Drawing for the job (mm, zero at the part's lowest x, y, z). Coordinates: 2 decimals unless noted, no trailing zeros. Order: outer loops, then holes, each group sorted by start corner. A loop starts at its lowest first (then second) coordinate and runs counter-clockwise, first axis right, second up.
1) Cut at A-A (y = 57.15). List the corners of the cut face in (x, z) (3 decimals), and give its area (3 significant figures).
2) Cut at D-D (z = 152). List the corners of the cut face in (x, y) (3 decimals).
3) Cut at B-B (z = 20). List the corners of the cut face in (x, y) (3 decimals).
4) Mould opens along X. For the marked faces 1, 2 and 3 say: +X half, -X half, draft (parallel to the pull), parting line (faces both ways), or undercut.
5) Pin check, flat tips, straight feed: pin 1 Ø1.5 at (y, z) = (34, 126.5) entering from -X; pin 2 Ø10 at (x, z) = (41, 117.5) entering from -Y; pin 3 Ø6 at (x, y) = (25, 43.5) entering from -Z; pin 4 Ø3 at (y, z) = (100.5, 117) entering from +X. Stop position of each tip, or through.
6) Wall check: L1, parallel to Y at x = 57, z = 135; L2, parallel to Z at x = 7, y = 31.5. Give the ranges that are in metal, low to high.
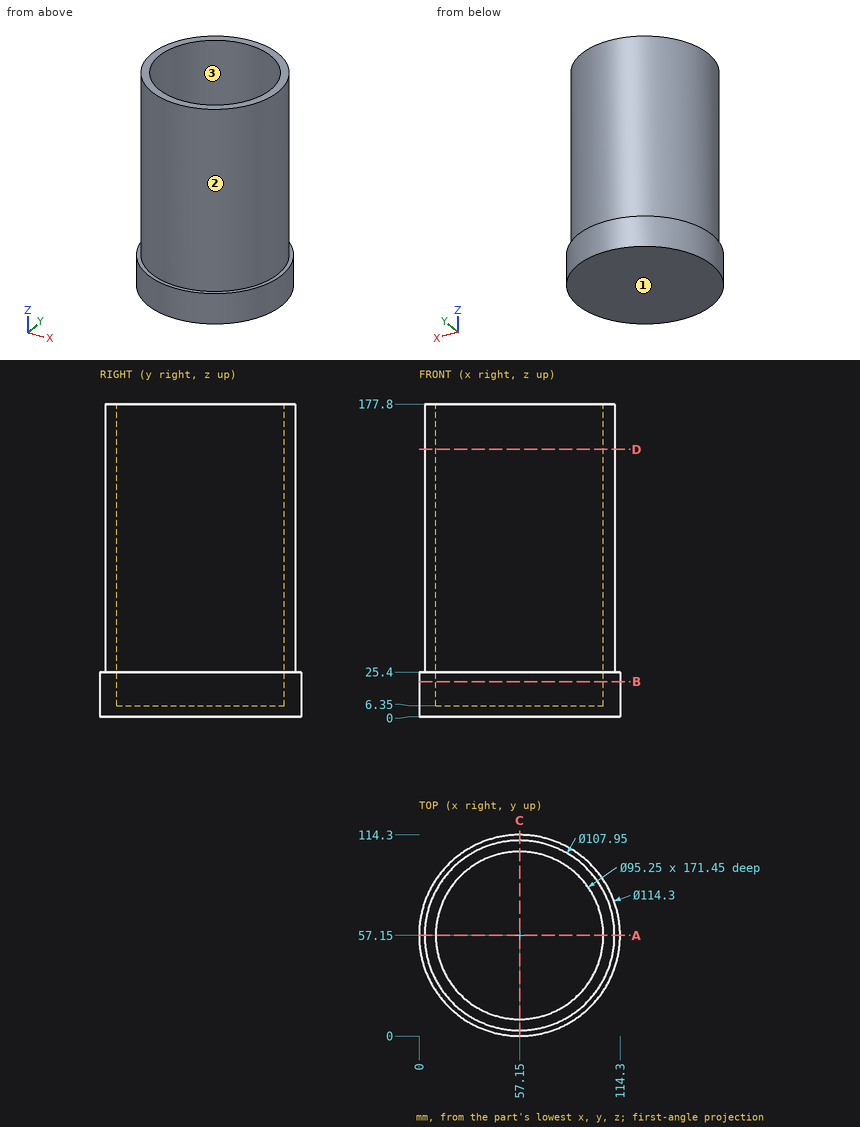
Geometry check:
1. outline: (0, 0) - (114.3, 0) - (114.3, 25.4) - (111.125, 25.4) - (111.125, 177.8) - (104.775, 177.8) - (104.775, 6.35) - (9.525, 6.35) - (9.525, 177.8) - (3.175, 177.8) - (3.175, 25.4) - (0, 25.4) - close
1. area: 3,020 mm2
2. outline: circle Ø107.95 at (57.15, 57.15); hole circle Ø95.25 at (57.15, 57.15)
3. outline: circle Ø114.3 at (57.15, 57.15); hole circle Ø95.25 at (57.15, 57.15)
4. face 1: draft
4. face 2: parting line
4. face 3: undercut
5. pin 1: stops at x = 8.04
5. pin 2: stops at y = 4.34
5. pin 3: stops at z = 0
5. pin 4: stops at x = 91.24
6. L1: y = 3.18 to 9.53, 104.77 to 111.12
6. L2: z = 0 to 25.4
